Geometry: final body of the model. Coordinates: model frame, mm. A direction names the side the tool comes from. Give positions to 0.01 mm unless a question says otherwise; leave off trailing zeros. Write each loop counter-clockwise with the first axis right and the second up, starting at its lowest first coordinate (ties: lowest second). Pieces come first, ordered by that corner, then holes. Notation, with made-up numbers: (12.25, 25.5) -> (51.25, 25.5) arc R22 cw to (51.25, 58.5) -> close; hole circle Ø9 at (49.25, 87.25). An arc over 180 degrees is marked (long way). Answer in a Markdown table with one row per item. Add a question column.
Item 1: Section query A-A on x = -16. Output: boundary loops of the cut face in (y, z).
Item 2: Material intervals for probe 1 along X at (y, z) = (15, -65); probe 2 along X at (y, z) = (27, -71); probe 3 along Z at (x, y) = (51, 45.5), sorted ascending. Write a range as from..to.
Item 3: Section query B-B on y = 31. Output: boundary loops of the cut face in (x, z), plus the area to 3 significant figures.
Item 4: First-contact query: P1, Ø3.5, axis at x = 21.9, z = 56.03, coming from the +Y side. Flat tip, straight axial feed; report the tip coordinate or a pass-through.
Item 5: Draft query along Y for faces 1 (the cylindrical face through (17.84, 26.7, 77.46)), 2 (the flat face through (-1, 20, -1)), 3 (the cylindrical face through (-2.65, 15.07, -21.14)). Return one class per face: +Y half, -Y half, draft (parallel to the pull), parting line (faces both ways), or undercut.
Item 6: Section query D-D on x = 27.5. Output: boundary loops of the cut face in (y, z), plus the area to 3 significant figures.
Item 7: Section query C-C on z = -60. Output: boundary loops of the cut face in (x, y), plus the area to 3 significant figures.
Item 8: Access query for faces 4 (the flat face through (1, 35, -80)), 5 (the flat face through (-55, 40, -1)). Directions: +Z, -Z, +X, -X, +Y, -Y. A direction counts if a zero-diameter tool reaches every point of the face in a straight line with its end or side. Return the directions, or none.
Autodesk Inventor part; units mm, degrees
ref_plane "YZ Plane" through (0, 0, 0) normal (1, 0, 0) x (0, 1, 0)
ref_plane "XZ Plane" through (0, 0, 0) normal (0, 1, 0) x (-1, 0, 0)
ref_plane "XY Plane" through (0, 0, 0) normal (0, 0, 1) x (1, 0, 0)
sketch "스케치1" plane through (0, 0, 0) normal (0, 1, 0) x (-1, 0, 0)
  line L0 (60, 80) -> (-60, 80)
  line L1 (-60, 80) -> (-60, -80)
  line L2 (-60, -80) -> (60, -80)
  line L3 (60, -80) -> (60, 80)
  line L4 (60, 80) -> (-60, -80) construction
  line L5 (-60, 80) -> (60, -80) construction
  point P0 (0, 0)
  dimension "d0" = 120
  dimension "d1" = 160
extrude "돌출1" add sketch "스케치1" along normal blind 60
sketch "스케치2" plane through (0, 60, 0) normal (0, 1, 0) x (1, 0, 0)
  line L0 (60, -80) -> (60, 80)
  line L1 (60, 80) -> (-60, 80)
  line L2 (55, 102.1646) -> (-55, 102.1646)
  line L3 (-55, 102.1646) -> (-55, -89.711)
  line L4 (-55, -89.711) -> (55, -89.711)
  line L5 (55, -89.711) -> (55, 102.1646)
  line L6 (-60, 80) -> (-60, -80)
  point P0 (0, 0)
  point P1 (55, 80)
  point P2 (-55, 80)
  dimension "d6" = 5
  dimension "d7" = 5
extrude "돌출2" cut sketch "스케치2" against normal blind 40 contours L5 L4 L3 L1
sketch "스케치9" plane through (0, 20, 0) normal (0, 1, 0) x (1, 0, 0)
  line L0 (-28.9457, -70) -> (24.4543, -70)
  line L1 (24.4543, -70) -> (24.4543, -1.4)
  line L2 (24.4543, -1.4) -> (-28.9457, -1.4)
  line L3 (-28.9457, -1.4) -> (-28.9457, -70)
  line L4 (55, -80) -> (-55, -80)
  circle A0 centre (-26.3957, -54.7) radius 1.6
  circle A1 centre (21.9043, -56.03) radius 1.6
  circle A2 centre (16.8243, -3.95) radius 1.6
  circle A3 centre (-11.1057, -3.95) radius 1.6
  point P0 (0, 0)
  dimension "d42" = 53.4
  dimension "d43" = 68.6
  dimension "d44" = 10
  dimension "d45" = 3.2
  dimension "d46" = 15.3
  dimension "d47" = 2.55
  dimension "d51" = 3.2
  dimension "d52" = 2.55
  dimension "d56" = 13.97
  dimension "d57" = 3.2
  dimension "d58" = 7.63
  dimension "d59" = 2.55
  dimension "d60" = 3.2
  dimension "d61" = 2.55
  dimension "d62" = 35.56
extrude "돌출8" cut sketch "스케치9" against normal through all contours A0 | A1 | A2 | A3
sketch "스케치12" plane through (60, 0, -80) normal (0, 0, -1) x (-1, 0, 0)
  line L0 (-34.8463, 10) -> (156.2634, 10)
  line L1 (156.2634, 10) -> (156.2634, -36.9465)
  line L2 (156.2634, -36.9465) -> (-34.8463, -36.9465)
  line L3 (-34.8463, -36.9465) -> (-34.8463, 10)
  line L4 (0, 0) -> (120, 0)
  point P0 (60, 0)
  dimension "d85" = 10
extrude "돌출10" cut sketch "스케치12" against normal through all
sketch "스케치13" plane through (-55, 20, 80) normal (0, 0, 1) x (1, 0, 0)
  line L0 (0, 40) -> (0, 0)
  line L1 (0, 0) -> (110, 0)
  line L2 (0, 40) -> (110, 40)
  line L3 (110, 40) -> (110, 0)
  line L4 (110, 0) -> (0, 0)
  line L5 (0, 0) -> (0, 40)
  point P0 (55, -20)
extrude "돌출11" add sketch "스케치13" against normal blind 5
sketch "스케치14" plane through (55, 20, -80) normal (0, 0, -1) x (-1, 0, 0)
  line L0 (0, 0) -> (0, 40)
  line L1 (110, 0) -> (0, 0)
  line L2 (0, 40) -> (110, 40)
  line L3 (110, 40) -> (110, 0)
  line L4 (110, 0) -> (0, 0)
  line L5 (0, 0) -> (0, 40)
  point P0 (55, -20)
extrude "돌출12" add sketch "스케치14" against normal blind 5
sketch "스케치15" plane through (60, 60, -80) normal (0, 0, -1) x (-1, 0, 0)
  point P0 (60, -60)
sketch "스케치16" plane through (60, 60, -80) normal (0, 0, -1) x (-1, 0, 0)
  point P0 (60, -60)
sketch "스케치17" plane through (0, 20, 0) normal (0, 1, 0) x (1, 0, 0)
  line L0 (-2.3, 22.7) -> (40, 22.7)
  line L1 (40, 22.7) -> (40, 65)
  line L2 (40, 65) -> (-2.3, 65)
  line L3 (-2.3, 65) -> (-2.3, 22.7)
  line L4 (55, 75) -> (55, -75)
  line L5 (55, 75) -> (-55, 75)
  circle A0 centre (-2.3, 22.7) radius 1.6
  circle A1 centre (-2.3, 65) radius 1.6
  circle A2 centre (40, 65) radius 1.6
  circle A3 centre (40, 22.7) radius 1.6
  line L6 (-47.9371, 14.7215) -> (-7.9371, 14.7215)
  line L7 (-7.9371, 14.7215) -> (-7.9371, 64.7215)
  line L8 (-7.9371, 64.7215) -> (-47.9371, 64.7215)
  line L9 (-47.9371, 64.7215) -> (-47.9371, 14.7215)
  point P0 (0, 0)
  dimension "d92" = 42.3
  dimension "d93" = 42.3
  dimension "d95" = 15
  dimension "d96" = 10
  dimension "d97" = 3.2
  dimension "d98" = 3.2
  dimension "d99" = 3.2
  dimension "d100" = 3.2
  dimension "d113" = 40
  dimension "d114" = 50
extrude "돌출13" cut sketch "스케치17" against normal through all contours L3 A0 L0 | L0 A0 L3 | A3 L1 L0 | L0 L1 A3 | A1 L2 L3 | L3 L2 A1 | A2 L2 L1 | L1 L2 A2
sketch "스케치19" plane through (60, 60, -80) normal (0, 0, -1) x (-1, 0, 0)
  line L0 (5, -40) -> (115, -40)
  circle A0 centre (44, -25) radius 8.5
  circle A1 centre (76, -25) radius 8.5
  line L1 (5, 0) -> (5, -40)
  line L2 (115, -40) -> (115, 0)
  point P0 (60, -60)
  dimension "d105" = 32
  dimension "d106" = 39
  dimension "d107" = 17
  dimension "d108" = 17
  dimension "d109" = 15
  dimension "d110" = 15
extrude "돌출14" cut sketch "스케치19" against normal through all
sketch "스케치21" plane through (0, 20, 0) normal (0, 1, 0) x (1, 0, 0)
  circle A0 centre (1.1314, 9.3126) radius 7.5
  line L0 (-49.3888, 17.2731) -> (-9.3888, 17.2731)
  line L1 (-9.3888, 17.2731) -> (-9.3888, 67.2731)
  line L2 (-9.3888, 67.2731) -> (-49.3888, 67.2731)
  line L3 (-49.3888, 67.2731) -> (-49.3888, 17.2731)
  point P0 (0, 0)
  dimension "d117" = 15
  dimension "d118" = 50
  dimension "d119" = 40
extrude "돌출15" cut sketch "스케치21" against normal through all contours A0
properties part number "본체판"
Findings below:
| question | item | result |
|---|---|---|
| 1 | outline | (10, -80) -> (26.5, -80) -> (26.5, -75) -> (20, -75) -> (20, 75) -> (26.5, 75) -> (26.5, 80) -> (10, 80) -> close; (43.5, -80) -> (60, -80) -> (60, -75) -> (43.5, -75) -> close; (43.5, 75) -> (60, 75) -> (60, 80) -> (43.5, 80) -> close |
| 2 | probe 1 | x = -60..-3.9, -0.7..38.4, 41.6..60 |
| 2 | probe 2 | x = -60..-55, 55..60 |
| 2 | probe 3 | z = -80..-75, 75..80 |
| 3 | outline | (-60, -80) -> (-23.5, -80) -> (-23.5, -75) -> (-55, -75) -> (-55, 75) -> (-23.5, 75) -> (-23.5, 80) -> (-60, 80) -> close; (-8.5, -80) -> (8.5, -80) -> (8.5, -75) -> (-8.5, -75) -> close; (-8.5, 75) -> (8.5, 75) -> (8.5, 80) -> (-8.5, 80) -> close; (23.5, -80) -> (60, -80) -> (60, 80) -> (23.5, 80) -> (23.5, 75) -> (55, 75) -> (55, -75) -> (23.5, -75) -> close |
| 3 | area | 2,400 mm^2 |
| 4 | P1 | stops at y = 20 |
| 5 | face 1 | undercut |
| 5 | face 2 | +Y half |
| 5 | face 3 | draft |
| 6 | outline | (10, -80) -> (60, -80) -> (60, -75) -> (20, -75) -> (20, 75) -> (60, 75) -> (60, 80) -> (10, 80) -> close |
| 6 | area | 2,000 mm^2 |
| 7 | outline | (-60, 10) -> (60, 10) -> (60, 60) -> (55, 60) -> (55, 20) -> (-55, 20) -> (-55, 60) -> (-60, 60) -> close |
| 7 | area | 1,600 mm^2 |
| 8 | face 4 | -Z, +X, -X, +Y, -Y |
| 8 | face 5 | +Y |
